```python
from build123d import *

# Parameters (mm, degrees)
SKETCH3_R                = 20
SKETCH3_R_2              = 10
BOSS_EXTRUDE4_DEPTH      = 40
SKETCH3_7_R              = 20
BOSS_EXTRUDE5_DEPTH      = 15
SKETCH3_8_W              = 65
SKETCH3_8_H              = 15
BOSS_EXTRUDE6_DEPTH      = 15
BOSS_EXTRUDE6_DEPTH_BACK = 15


with BuildPart() as part:
    # Sketch3 → Boss-Extrude4 (new body)
    with BuildSketch(Plane(origin=(0, 0, 0), x_dir=(1, 0, 0), z_dir=(0, 1, 0))):
        Circle(SKETCH3_R)
        Circle(SKETCH3_R_2, mode=Mode.SUBTRACT)
    extrude(amount=BOSS_EXTRUDE4_DEPTH)

    # Sketch3_7 → Boss-Extrude5 (add)
    with BuildSketch(Plane(origin=(0, 0, 0), x_dir=(1, 0, 0), z_dir=(0, 1, 0))):
        with BuildLine():
            Line((32.5, 53), (-32.5, 53))
            Line((-32.5, 53), (-32.5, 0))
            ThreePointArc((-32.5, 0), (0, -32.5), (32.5, 0))
            Line((32.5, 0), (32.5, 53))
        make_face()
        Circle(SKETCH3_7_R, mode=Mode.SUBTRACT)
    extrude(amount=BOSS_EXTRUDE5_DEPTH)

    # Sketch3_8 → Boss-Extrude6 (add, two sides)
    with BuildSketch(Plane(origin=(0, 0, 0), x_dir=(1, 0, 0), z_dir=(0, 1, 0))) as boss_extrude6_sk:
        with Locations((0, 60.5)):
            Rectangle(SKETCH3_8_W, SKETCH3_8_H)
    extrude(amount=BOSS_EXTRUDE6_DEPTH)
    extrude(boss_extrude6_sk.sketch, amount=-BOSS_EXTRUDE6_DEPTH_BACK)


solid = part.part
```
For this review, take the finished solid that the model builds, in its own axes (mm). A direction names the side the tool comes from. Round coordinates to 2 decimals unless told otherwise and drop trailing zeros. Loops run counter-clockwise (first coordinate to the right, second up) from the corner with the lowest first, then second, coordinate; pieces in that order, holes last.
(1) Mouldability with a two-part tool opening along X and no side actions: class faces 3 (the cylindrical face through (-2.17, 19.72, 9.76)), 4 (the cylindrical face through (-4.336, 27.325, 19.524)), 5 (the flat face through (0, 0, -68)) as released by +X, released by -X, zero draft, split by the parting line, or undercut.
Returned:
face 3: undercut
face 4: split by the parting line
face 5: zero draft
(2) Tool access review of faces 1 (the flat face through (0, -7, -53)), 2 (the flat face through (-32.5, 4, -41)): name each direction out of +Z, -Z, +X, -X, +Y, -Y from which nothing blocks a thin tool from reaching the whole face with its end or side.
Returned:
face 1: +Z, +X, -X, -Y
face 2: +Z, -Z, -X, +Y, -Y
(3) We need section C-C (y = 11). Give the boundary of the cut face in (x, z), plus the area to 4 significant figures.
Returned:
outline: (-32.5, -68) - (32.5, -68) - (32.5, 0) arc R32.5 ccw to (-32.5, 0) - close; hole circle Ø20 at (0, 0)
area: 5,765 mm2
(4) We need section D-D (z = -25). Give the boundary of the cut face in (x, y), plus the area to 3 significant figures.
Returned:
outline: (-32.5, 0) - (32.5, 0) - (32.5, 15) - (-32.5, 15) - close
area: 975 mm2
(5) Wall thickness on line 1 along Z through (x, y) = (0, 32); line 2 along Z through (x, y) = (0, 13.5); line 3 along X through (y, z) = (14.5, 0.5): over which ranges is each line inside the solid? List them lowest first.
Returned:
line 1: z = -20 to -10, 10 to 20
line 2: z = -68 to -10, 10 to 32.5
line 3: x = -32.5 to -9.99, 9.99 to 32.5
(6) We need section A-A (x = 0). Give the boundary of the cut face in (y, z).
Returned:
outline: (-15, -68) - (15, -68) - (15, -20) - (40, -20) - (40, -10) - (0, -10) - (0, -53) - (-15, -53) - close; (0, 10) - (40, 10) - (40, 20) - (15, 20) - (15, 32.5) - (0, 32.5) - close
(7) Clearance check with flat-ended pins moving along their axes: P1, Ø8, axis at x = -16.5, z = -22.5, coming from the -Y side; P2, Ø12, axis at x = 3, y = -8.5, coming from the +Z side; P3, Ø1.5, axis at x = 20.5, y = 0.5, coming from the +Z side. State where each tip first meets the part, or that it passes through.
Returned:
P1: stops at y = 0
P2: stops at z = -53
P3: stops at z = 25.81
(8) We need section B-B (z = -8). Give the boundary of the cut face in (x, y), plus the area to 3 significant figures.
Returned:
outline: (-32.5, 0) - (-6, 0) - (-6, 40) - (-18.33, 40) - (-18.33, 15) - (-32.5, 15) - close; (6, 0) - (32.5, 0) - (32.5, 15) - (18.33, 15) - (18.33, 40) - (6, 40) - close
area: 1,410 mm2
